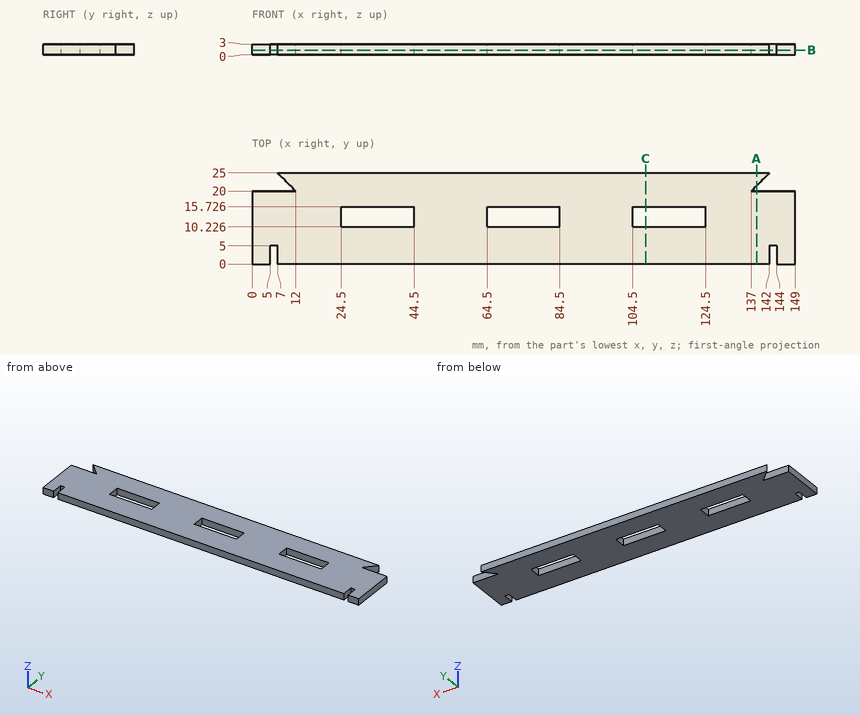
Can you work these out from the drawing? Everything is in mm from the part's minimum corner. Give positions to 0.01 mm unless a question says otherwise; leave off trailing zeros. Order: outer loops, then holes, each group sorted by start corner. A loop starts at its lowest first (then second) coordinate and runs counter-clockwise, first axis right, second up.
Item 1: If we section it at B-B, the plane z = 1.35: Write out the boundary of the cut face in (x, y) (1 decimal).
Item 2: If we section it at C-C, the plane x = 108: Write out the boundary of the cut face in (y, z) (1 decimal), plus the area to 3 significant figures.
Item 3: I need wall thicknesses on line 1 (X direction, y = 10.75, z = 2.1); line 2 (X direction, y = 2, z = 0.35); line 3 (Y direction, x = 121.5, z = 2.65) (1 decimal). Which ranges of each line are inside material? Lowest first, please.
Item 4: If we section it at A-A, the plane x = 138.5: Write out the boundary of the cut face in (y, z).
Item 5: I'm going to push a flat-ended pin straight in: pin 1 (1.6 mm diameter, centred on x = 143, z = 2, fed in from -Y). Where does the tip first touch, or does it pass through?
Values:
1. outline: (0, 0) - (5, 0) - (5, 5) - (7, 5) - (7, 0) - (142, 0) - (142, 5) - (144, 5) - (144, 0) - (149, 0) - (149, 20) - (137, 20) - (142, 25) - (7, 25) - (12, 20) - (0, 20) - close; hole (24.5, 10.2) - (44.5, 10.2) - (44.5, 15.7) - (24.5, 15.7) - close; hole (64.5, 10.2) - (84.5, 10.2) - (84.5, 15.7) - (64.5, 15.7) - close; hole (104.5, 10.2) - (124.5, 10.2) - (124.5, 15.7) - (104.5, 15.7) - close
2. outline: (0, 0) - (10.2, 0) - (10.2, 3) - (0, 3) - close; (15.7, 0) - (25, 0) - (25, 3) - (15.7, 3) - close
2. area: 58.5 mm2
3. line 1: x = 0 to 24.5, 44.5 to 64.5, 84.5 to 104.5, 124.5 to 149
3. line 2: x = 0 to 5, 7 to 142, 144 to 149
3. line 3: y = 0 to 10.2, 15.7 to 25
4. outline: (0, 0) - (20, 0) - (20, 3) - (0, 3) - close; (21.5, 0) - (25, 0) - (25, 3) - (21.5, 3) - close
5. pin 1: stops at y = 5
